```python
from build123d import *

# Parameters (mm, degrees)
SKETCH1_W               = 50
SKETCH1_H               = 50
BOSS_EXTRUDE1_DEPTH     = 75
FILLET1_R               = 5
SKETCH2_W               = 42.5
SKETCH2_H               = 42.5
CUT_EXTRUDE1_DEPTH      = 70
FILLET2_R               = 3
SKETCH3_W               = 25.5
SKETCH3_H               = 3.75
SKETCH3_W_2             = 3.75
SKETCH3_H_2             = 25.5
CUT_EXTRUDE2_DEPTH      = 50
SKETCH4_W               = 20
SKETCH4_H               = 3.75
CUT_EXTRUDE3_DEPTH      = 70
BOSS_EXTRUDE2_DEPTH     = 20
SKETCH6_W               = 40
SKETCH6_H               = 10
BOSS_EXTRUDE4_DEPTH     = 75
SKETCH7_W               = 7
SKETCH7_H               = 20
CUT_EXTRUDE4_DEPTH      = 8
SKETCH8_R               = 1.55
CUT_EXTRUDE5_DEPTH      = 5
SKETCH9_R               = 4
CUT_EXTRUDE6_DEPTH      = 5
MIRROR2_COPY_1_SKETCH_R = 1.55
MIRROR2_COPY_1_DEPTH    = 5
MIRROR2_COPY_2_SKETCH_R = 4
MIRROR2_COPY_2_DEPTH    = 5
SKETCH11_W              = 40
SKETCH11_H              = 10
BOSS_EXTRUDE5_DEPTH     = 10
SKETCH12_R              = 4
CUT_EXTRUDE7_DEPTH      = 46
SKETCH13_R              = 16.25
CUT_EXTRUDE8_DEPTH      = 5
SKETCH14_R              = 16.25
CUT_EXTRUDE9_DEPTH      = 12
SKETCH15_R              = 8.1
CUT_EXTRUDE10_DEPTH     = 12
SKETCH16_R              = 2
CUT_EXTRUDE11_DEPTH     = 12
SKETCH17_W              = 7
SKETCH17_H              = 20
CUT_EXTRUDE12_DEPTH     = 20
SKETCH18_W              = 65
SKETCH18_H              = 28
BOSS_EXTRUDE6_DEPTH     = 10
SKETCH19_W              = 14
SKETCH19_H              = 6
CUT_EXTRUDE13_DEPTH     = 130
SKETCH20_W              = 7
SKETCH20_H              = 20
CUT_EXTRUDE14_DEPTH     = 3


with BuildPart() as part:
    # Sketch1 → Boss-Extrude1 (new body)
    with BuildSketch(Plane(origin=(0, 0, 0), x_dir=(0, 0, -1), z_dir=(1, 0, 0))):
        Rectangle(SKETCH1_W, SKETCH1_H)
    extrude(amount=-BOSS_EXTRUDE1_DEPTH)

    # Fillet1
    fillet1_edges = [part.edges().sort_by_distance(p)[0] for p in [
        (-37.5, -25, -25),
        (-37.5, -25, 25),
        (-37.5, 25, 25),
        (-37.5, 25, -25),
    ]]
    fillet(fillet1_edges, radius=FILLET1_R)

    # Sketch2 → Cut-Extrude1 (cut)
    with BuildSketch(Plane(origin=(0, 0, 0), x_dir=(0, 0, -1), z_dir=(1, 0, 0))):
        Rectangle(SKETCH2_W, SKETCH2_H)
    extrude(amount=-CUT_EXTRUDE1_DEPTH, mode=Mode.SUBTRACT)

    # Fillet2
    fillet2_edges = [part.edges().sort_by_distance(p)[0] for p in [
        (-35, 21.25, -21.25),
        (-35, -21.25, -21.25),
        (-35, -21.25, 21.25),
        (-35, 21.25, 21.25),
    ]]
    fillet(fillet2_edges, radius=FILLET2_R)

    # Sketch3 → Cut-Extrude2 (cut)
    with BuildSketch(Plane(origin=(0, 0, 0), x_dir=(0, 0, -1), z_dir=(1, 0, 0))):
        with Locations((0, 23.125)):
            Rectangle(SKETCH3_W, SKETCH3_H)
        with Locations((-23.125, 0)):
            Rectangle(SKETCH3_W_2, SKETCH3_H_2)
        with Locations((23.125, 0)):
            Rectangle(SKETCH3_W_2, SKETCH3_H_2)
    extrude(amount=-CUT_EXTRUDE2_DEPTH, mode=Mode.SUBTRACT)

    # Sketch4 → Cut-Extrude3 (cut)
    with BuildSketch(Plane(origin=(0, 0, 0), x_dir=(0, 0, -1), z_dir=(1, 0, 0))):
        with Locations((0, -23.125)):
            Rectangle(SKETCH4_W, SKETCH4_H)
    extrude(amount=-CUT_EXTRUDE3_DEPTH, mode=Mode.SUBTRACT)



with BuildPart() as body_2:
    # Sketch5 → Boss-Extrude2 (new body)
    with BuildSketch(Plane.XZ.offset(25)):
        Polygon((15, 20), (0, 20), (0, 10), (0, -10), (0, -20), (15, -20), align=None)
        with BuildLine():
            ThreePointArc((15, 20), (35, 0), (15, -20))
            Line((15, -20), (15, 20))
        make_face()
    extrude(amount=BOSS_EXTRUDE2_DEPTH)


with BuildPart() as part_1:
    add(part.part)

    add(body_2.part)  # Boss-Extrude4 merges body 2
    # Sketch6 → Boss-Extrude4 (add)
    with BuildSketch(Plane.ZY):
        with Locations((0, -30)):
            Rectangle(SKETCH6_W, SKETCH6_H)
    extrude(amount=BOSS_EXTRUDE4_DEPTH)

    # Sketch7 → Cut-Extrude4 (cut)
    with BuildSketch(Plane(origin=(0, -25, 0), x_dir=(1, 0, 0), z_dir=(0, 1, 0))):
        with Locations((-66.5, 0)):
            Rectangle(SKETCH7_W, SKETCH7_H)
    extrude(amount=-CUT_EXTRUDE4_DEPTH, mode=Mode.SUBTRACT)

    # Sketch8 → Cut-Extrude5 (cut)
    with BuildSketch(Plane(origin=(0, 0, 0), x_dir=(0, 0, -1), z_dir=(1, 0, 0))):
        with Locations((-22, 21.6)):
            Circle(SKETCH8_R)
    cut_extrude5 = extrude(amount=-CUT_EXTRUDE5_DEPTH, mode=Mode.SUBTRACT)

    # Sketch9 → Cut-Extrude6 (cut)
    with BuildSketch(Plane(origin=(-5, 0, 0), x_dir=(0, 0, -1), z_dir=(1, 0, 0))):
        with Locations((-22, 21.6)):
            Circle(SKETCH9_R)
    cut_extrude6 = extrude(amount=-CUT_EXTRUDE6_DEPTH, mode=Mode.SUBTRACT)

    # Mirror1: Cut-Extrude5, Cut-Extrude6 across plane
    add(cut_extrude5.mirror(Plane.ZX), mode=Mode.SUBTRACT)
    add(cut_extrude6.mirror(Plane.ZX), mode=Mode.SUBTRACT)

    # Mirror2: Cut-Extrude5, Cut-Extrude6 across plane
    add(cut_extrude5.mirror(Plane.XY), mode=Mode.SUBTRACT)
    add(cut_extrude6.mirror(Plane.XY), mode=Mode.SUBTRACT)

    # Mirror2 copy 1 sketch → Mirror2 copy 1 (cut)
    with BuildSketch(Plane(origin=(0, 0, 0), x_dir=(0, 0, 1), z_dir=(1, 0, 0))):
        with Locations((-22, 21.6)):
            Circle(MIRROR2_COPY_1_SKETCH_R)
    extrude(amount=-MIRROR2_COPY_1_DEPTH, mode=Mode.SUBTRACT)

    # Mirror2 copy 2 sketch → Mirror2 copy 2 (cut)
    with BuildSketch(Plane(origin=(-5, 0, 0), x_dir=(0, 0, 1), z_dir=(1, 0, 0))):
        with Locations((-22, 21.6)):
            Circle(MIRROR2_COPY_2_SKETCH_R)
    extrude(amount=-MIRROR2_COPY_2_DEPTH, mode=Mode.SUBTRACT)

    # Sketch11 → Boss-Extrude5 (add)
    with BuildSketch(Plane.ZY):
        with Locations((0, -40)):
            Rectangle(SKETCH11_W, SKETCH11_H)
    extrude(amount=BOSS_EXTRUDE5_DEPTH)

    # Sketch12 → Cut-Extrude7 (cut, through all)
    with BuildSketch(Plane.XY.offset(20)):
        with Locations((15, -35)):
            Circle(SKETCH12_R)
    extrude(amount=-CUT_EXTRUDE7_DEPTH, mode=Mode.SUBTRACT)

    # Sketch13 → Cut-Extrude8 (cut)
    with BuildSketch(Plane(origin=(0, -25, 0), x_dir=(1, 0, 0), z_dir=(0, 1, 0))):
        with Locations((15, 0)):
            Circle(SKETCH13_R)
    extrude(amount=-CUT_EXTRUDE8_DEPTH, mode=Mode.SUBTRACT)

    # Sketch14 → Cut-Extrude9 (cut)
    with BuildSketch(Plane.XZ.offset(45)):
        with Locations((15, 0)):
            Circle(SKETCH14_R)
    extrude(amount=-CUT_EXTRUDE9_DEPTH, mode=Mode.SUBTRACT)

    # Sketch15 → Cut-Extrude10 (cut)
    with BuildSketch(Plane(origin=(0, -30, 0), x_dir=(1, 0, 0), z_dir=(0, 1, 0))):
        with Locations((15, 0)):
            Circle(SKETCH15_R)
    extrude(amount=-CUT_EXTRUDE10_DEPTH, mode=Mode.SUBTRACT)

    # Sketch16 → Cut-Extrude11 (cut)
    with BuildSketch(Plane.XZ.offset(33)):
        with Locations((6.514718626, 8.485281374)):
            Circle(SKETCH16_R)
        with Locations((23.485281374, 8.485281374)):
            Circle(SKETCH16_R)
        with Locations((23.485281374, -8.485281374)):
            Circle(SKETCH16_R)
        with Locations((6.514718626, -8.485281374)):
            Circle(SKETCH16_R)
    extrude(amount=-CUT_EXTRUDE11_DEPTH, mode=Mode.SUBTRACT)

    # Sketch17 → Cut-Extrude12 (cut)
    with BuildSketch(Plane(origin=(0, -33, 0), x_dir=(1, 0, 0), z_dir=(0, 1, 0))):
        with Locations((-66.5, 0)):
            Rectangle(SKETCH17_W, SKETCH17_H)
    extrude(amount=-CUT_EXTRUDE12_DEPTH, mode=Mode.SUBTRACT)

    # Sketch18 → Boss-Extrude6 (add)
    with BuildSketch(Plane.XZ.offset(35)):
        with Locations((-42.5, 0)):
            Rectangle(SKETCH18_W, SKETCH18_H)
    extrude(amount=BOSS_EXTRUDE6_DEPTH)

    # Sketch19 → Cut-Extrude13 (cut)
    with BuildSketch(Plane.ZY.offset(75)):
        with Locations((0, -40)):
            Rectangle(SKETCH19_W, SKETCH19_H)
    extrude(amount=-CUT_EXTRUDE13_DEPTH, mode=Mode.SUBTRACT)

    # Sketch20 → Cut-Extrude14 (cut)
    with BuildSketch(Plane(origin=(0, -35, 0), x_dir=(1, 0, 0), z_dir=(0, 1, 0))):
        with Locations((-66.5, 0)):
            Rectangle(SKETCH20_W, SKETCH20_H)
    extrude(amount=-CUT_EXTRUDE14_DEPTH, mode=Mode.SUBTRACT)


solid = part_1.part
```
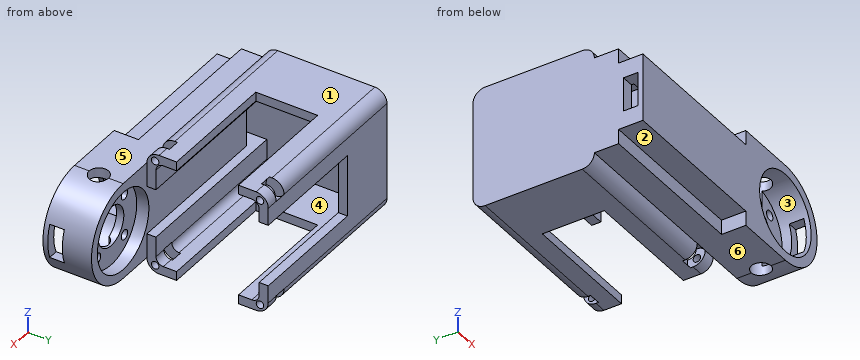
Can you work these out from the model? Positions are in its coordinate system, mm. Face numbers are marked on the shaded views. A direction names the side the tool comes from. Give positions to 0.01 mm unless a question says otherwise; leave off trailing zeros. Order: outer loops, then holes, each group sorted by start corner. A loop starts at its lowest first (then second) coordinate and runs counter-clockwise, first axis right, second up. Notation, with made-up numbers: (-30, -12.5) - (3, -12.5) arc R34 cw to (3, 21.5) - close; hole circle Ø9 at (72, -20.5). An arc over 180 degrees is marked (long way). Use a Markdown table: item, result. Add a question column.
Q1. Please list where these lines run through material, in increasing order: line 1 along X through (y, z) = (-28.9, 0); line 2 along Y through (x, z) = (-3, -22); line 3 along Z through (x, y) = (-43.5, 14.5).
Q2. On a 3-axis mill with a long thin cutter (end or side, diameter ignored), from which of +Z, -Z, +X, -X, +Y, -Y can I reach the whole of each face in a straight line? I mean the marked faces 4, 5 and 6. Say none if no direction works.
Q3. I'm going to push flat-ended pins straight in: pin 1 (21 mm diameter, centred on x = 15, z = 0, fed in from +Y); pin 2 (6 mm diameter, centred on y = -37.5, z = -6.5, fed in from +X); pin 3 (8 mm diameter, centred on x = -3.5, y = -35.5, fed in from -Z). Where does each tip first touch, or does it pass through?
Q4. If we section it at A-A on x = -19: Count the separate pieces of the cut face and the enclosed holes in it, plus the area to 3 significant figures.
Q5. If we mould it in two halves opening along Z, with no side actions, what happens to the marked faces 1, 2 and 3? For each: released by +Z, released by -Z, zero draft, split by the parting line, or undercut.
Q6. If we section it at B-B on y = -8: Write out the boundary of the cut face in (x, z), plus the area to 3 significant figures.
Answers follow:
| question | item | result |
|---|---|---|
| 1 | line 1 | x = -75 to -70, -63 to -1.25, 31.25 to 35 |
| 1 | line 2 | y = -24.58 to -23.15, -20.05 to -12.75, 12.75 to 20.05, 23.15 to 24.58 |
| 1 | line 3 | z = -25 to -21.25, 21.25 to 25 |
| 2 | face 4 | +X |
| 2 | face 5 | +Z, +X, -X, -Y |
| 2 | face 6 | -Z, +X, -X, -Y |
| 3 | pin 1 | stops at y = -30 |
| 3 | pin 2 | stops at x = 34.68 |
| 3 | pin 3 | stops at z = -20 |
| 4 | separate pieces | 3 |
| 4 | enclosed holes | 1 |
| 4 | area | 914 mm^2 |
| 5 | face 1 | released by +Z |
| 5 | face 2 | released by -Z |
| 5 | face 3 | undercut |
| 6 | outline | (-75, -25) - (-50, -25) - (-50, -21.25) - (-70, -21.25) - (-70, 21.25) - (-50, 21.25) - (-50, 25) - (-75, 25) - close |
| 6 | area | 400 mm^2 |
